from build123d import *

# Parameters (mm, degrees)
F1_DEPTH = 2.5
F2_R     = 2.5
F3_DEPTH = 25


with BuildPart() as f1:
    # F0 (on Top) → F1 (new body)
    with BuildSketch(Plane.XY):
        with BuildLine():
            ThreePointArc((3.5, -3.5), (5.9748737342, -2.4748737342), (7, 0))
            ThreePointArc((7, 0), (5.9748737342, 2.4748737342), (3.5, 3.5))
            Line((3.5, 3.5), (3.5, -3.5))
        make_face()
        with BuildLine():
            ThreePointArc((-3.5, -3.5), (-1.0251262658, -2.4748737342), (0, 0))
            ThreePointArc((0, 0), (-1.0251262658, 2.4748737342), (-3.5, 3.5))
            ThreePointArc((-3.5, 3.5), (-7, 0), (-3.5, -3.5))
        make_face()
        with BuildLine():
            ThreePointArc((0, 0), (1.0251262658, 2.4748737342), (3.5, 3.5))
            Line((3.5, 3.5), (0, 3.5))
            Line((0, 3.5), (0, 0))
        make_face()
        with BuildLine():
            Line((3.5, -3.5), (3.5, 3.5))
            ThreePointArc((3.5, 3.5), (1.0251262658, 2.4748737342), (0, 0))
            ThreePointArc((0, 0), (1.0251262658, -2.4748737342), (3.5, -3.5))
        make_face()
        with BuildLine():
            ThreePointArc((-3.5, 3.5), (-1.0251262658, 2.4748737342), (0, 0))
            Line((0, 0), (0, 3.5))
            Line((0, 3.5), (-3.5, 3.5))
        make_face()
        with BuildLine():
            Line((0, -3.5), (0, 0))
            ThreePointArc((0, 0), (-1.0251262658, -2.4748737342), (-3.5, -3.5))
            Line((-3.5, -3.5), (0, -3.5))
        make_face()
        with BuildLine():
            Line((0, -3.5), (3.5, -3.5))
            ThreePointArc((3.5, -3.5), (1.0251262658, -2.4748737342), (0, 0))
            Line((0, 0), (0, -3.5))
        make_face()
    extrude(amount=F1_DEPTH)

    # F2 (on face) → F3 (cut)
    with BuildSketch(Plane.XY.offset(2.5)):
        with Locations((-3.5, 0)):
            Circle(F2_R)
        with Locations((3.5, 0)):
            Circle(F2_R)
    extrude(amount=-F3_DEPTH, mode=Mode.SUBTRACT)


solid = f1.part
Verification items for the finished model (mm, model axes). Give positions to 0.01 mm unless a question says otherwise; leave off trailing zeros. Loops run counter-clockwise (first coordinate to the right, second up) from the corner with the lowest first, then second, coordinate; pieces in that order, holes last.
1. Cross-section at D-D on x = -4. Record the cut outline in (y, z), and give its area (3 significant figures).
Derived:
outline: (-3.46, 0) - (-2.45, 0) - (-2.45, 2.5) - (-3.46, 2.5) - close; (2.45, 0) - (3.46, 0) - (3.46, 2.5) - (2.45, 2.5) - close
area: 5.07 mm2
2. Release check for a two-part mould opening along Y. For faces 1 (the flat face through (0, -3.5, 1)), 2 (the cylindrical face through (5.885, 0.751, 1.268)), 3 (the cylindrical face through (-7, 0, 1)), 4 (the flat face through (0, 0, 2.5)) record: +Y half, -Y half, draft (parallel to the pull), parting line (faces both ways), or undercut.
Derived:
face 1: -Y half
face 2: undercut
face 3: parting line
face 4: draft
3. Material ranges on probe 1 along Y at (x, z) = (-3.5, 1.4); probe 2 along X at (y, z) = (-1.5, 1.1); probe 3 along X at (y, z) = (0.5, 1.5), recorded low to high.
Derived:
probe 1: y = -3.5 to -2.5, 2.5 to 3.5
probe 2: x = -6.66 to -5.5, -1.5 to 1.5, 5.5 to 6.66
probe 3: x = -6.96 to -5.95, -1.05 to 1.05, 5.95 to 6.96
4. Cross-section at A-A on x = -1.5. Record the cut outline in (y, z).
Derived:
outline: (-3.5, 0) - (-1.5, 0) - (-1.5, 2.5) - (-3.5, 2.5) - close; (1.5, 0) - (3.5, 0) - (3.5, 2.5) - (1.5, 2.5) - close
5. Cross-section at C-C on y = -1.25. Record the cut outline in (x, z).
Derived:
outline: (-6.77, 0) - (-5.67, 0) - (-5.67, 2.5) - (-6.77, 2.5) - close; (-1.33, 0) - (1.33, 0) - (1.33, 2.5) - (-1.33, 2.5) - close; (5.67, 0) - (6.77, 0) - (6.77, 2.5) - (5.67, 2.5) - close
6. Cross-section at B-B on z = 2.25. Record the cut outline in (x, y), and give its area (3 significant figures).
Derived:
outline: (-3.5, -3.5) - (3.5, -3.5) arc R3.5 ccw to (3.5, 3.5) - (-3.5, 3.5) arc R3.5 ccw to start; hole circle Ø5 at (-3.5, 0); hole circle Ø5 at (3.5, 0)
area: 48.2 mm2
